from build123d import *

# Parameters (mm, degrees)
ESQUISSE2_R             = 3
ENL_V_MAT_EXTRU_1_DEPTH = 30.546573405
ESQUISSE3_R             = 1.5
ENL_V_MAT_EXTRU_2_DEPTH = 30.54657341


with BuildPart() as part:
    # Esquisse1 → Révolution1 (revolve)
    with BuildSketch(Plane.XY):
        with BuildLine():
            Line((0, 15), (0, -15))
            Line((0, -15), (-9.949874371, -15))
            ThreePointArc((-9.949874371, -15), (-18, 0), (-9.949874371, 15))
            Line((-9.949874371, 15), (0, 15))
        make_face()
    revolve(axis=Axis((0, 15, 0), (0, -1, 0)))

    # Esquisse2 → Enlèv. mat.-Extru.1 (cut, through all)
    with BuildSketch(Plane(origin=(0, 0, 0), x_dir=(0, 0, -1), z_dir=(1, 0, 0))):
        Circle(ESQUISSE2_R)
    extrude(amount=-ENL_V_MAT_EXTRU_1_DEPTH, mode=Mode.SUBTRACT)

    # Esquisse3 → Enlèv. mat.-Extru.2 (cut, through all)
    with BuildSketch(Plane(origin=(0, 0, 0), x_dir=(0, 0, -1), z_dir=(1, 0, 0))):
        with Locations((0, -10.5)):
            Circle(ESQUISSE3_R)
    extrude(amount=-ENL_V_MAT_EXTRU_2_DEPTH, mode=Mode.SUBTRACT)


solid = part.part
Input: part model. Units: mm. Frame: model coordinates. A direction names the side the tool comes from. Give positions to 0.01 mm unless a question says otherwise; leave off trailing zeros. Loops run counter-clockwise (first coordinate to the right, second up) from the corner with the lowest first, then second, coordinate; pieces in that order, holes last. Notation, with made-up numbers: (59.5, 32) -> (95.5, 32) arc R19 cw to (95.5, 44) -> close; hole circle Ø6 at (0, 82.25). An arc over 180 degrees is marked (long way). Answer as a JSON object with one key per item and string values. Group by question number.
Item 1: Cut plane A-A, the plane z = 0. Return the cut outline in (x, y).
Item 2: Reachability of faces 1 (the cylindrical face through (-8.75, 0.9, -2.86)), 2 (the flat face through (0, 15, 0)) from +Z, -Z, +X, -X, +Y, -Y: full face, straight path, thin tool, end or side. Return the list, or none.
Item 3: Pin query (flat end, axial travel): P1, Ø8, axis at x = -3, y = 5.5, coming from the +Z side; P2, Ø10, axis at x = -1.5, y = -4, coming from the +Z side; P3, Ø8, axis at x = 7, z = 12.5, coming from the -Y side; P4, Ø3, axis at y = -1.5, z = 1.5, coming from the -X side. Return the tip coordinate at first contact, or that it passes through.
Item 4: Cut plane C-C, the plane x = -12. Return the cut outline in (y, z), and give its area (3 significant figures).
Item 5: Pull-direction query (Z, two-part tool) for faces 3 (the flat face through (0, 0, 0)), 4 (the flat face through (0, -15, 0)); classes: released by +Z, released by -Z, zero draft, split by the parting line, or undercut.
Item 6: Cut plane B-B, the plane y = 0. Return the cut outline in (x, z).
Item 7: Cut plane D-D, the plane y = -13. Return the cut outline in (x, z).
Item 8: Line query: probe 1 along Y at (x, z) = (-5.5, 0); probe 2 along Z at (x, y) = (-10, 0); probe 3 along Y at (x, z) = (-1.5, 2.5). Output: solid intervals per line, ascending.
Checks:
{
 "1": {"outline": "(-17.75, -3) arc R18 ccw to (-15.59, -9) -> (0, -9) -> (0, -12) -> (-13.42, -12) arc R18 ccw to (-9.95, -15) -> (9.95, -15) arc R18 ccw to (9.95, 15) -> (-9.95, 15) arc R18 ccw to (-17.75, 3) -> (0, 3) -> (0, -3) -> close"},
 "2": {"face 1": "-X", "face 2": "+Z, -Z, +X, -X, +Y"},
 "3": {"P1": "stops at z = 17.86", "P2": "stops at z = 18", "P3": "stops at y = -14.74", "P4": "stops at x = -17.75"},
 "4": {"outline": "circle Ø26.83 at (0, 0); hole circle Ø3 at (-10.5, 0); hole circle Ø6 at (0, 0)", "area": "530 mm²"},
 "5": {"face 3": "undercut", "face 4": "zero draft"},
 "6": {"outline": "(-17.75, -3) arc R18 ccw (long way) to (-17.75, 3) -> (0, 3) -> (0, -3) -> close"},
 "7": {"outline": "circle Ø24.9 at (0, 0)"},
 "8": {"probe 1": "y = -15 to -12, -9 to -3, 3 to 15", "probe 2": "z = -14.97 to -3, 3 to 14.97", "probe 3": "y = -15 to -1.66, 1.66 to 15"}
}
